Autodesk Inventor part; units mm, degrees
ref_plane "YZ Plane" through (0, 0, 0) normal (1, 0, 0) x (0, 1, 0)
ref_plane "XZ Plane" through (0, 0, 0) normal (0, 1, 0) x (-1, 0, 0)
ref_plane "XY Plane" through (0, 0, 0) normal (0, 0, 1) x (1, 0, 0)
sketch "Sketch1" plane through (0, 0, 0) normal (0, 1, 0) x (-1, 0, 0)
  line L0 (0, 0) -> (0, -3)
  line L1 (-250, -38) -> (-250, -78)
  line L2 (0, 0) -> (-20, 0)
  line L3 (-50, 0) -> (-50, -3)
  line L4 (-50, 0) -> (-70, 0)
  line L5 (-70, 0) -> (-70, -3)
  line L6 (-100, 0) -> (-100, -3)
  line L7 (-100, 0) -> (-120, 0)
  line L8 (-120, 0) -> (-120, -3)
  line L9 (-150, 0) -> (-150, -3)
  line L10 (-150, 0) -> (-170, 0)
  line L11 (-170, 0) -> (-170, -3)
  line L12 (-200, 0) -> (-200, -3)
  line L13 (-200, 0) -> (-220, 0)
  line L14 (-220, 0) -> (-220, -3)
  line L15 (-20, 0) -> (-20, -3)
  line L16 (-250, -58) -> (-250, -78)
  line L17 (-250, -78) -> (-247, -78)
  line L18 (-247, -78) -> (-247, -113)
  line L19 (-250, -58) -> (-250, -38)
  line L20 (-250, -38) -> (-247, -38)
  line L21 (-247, -38) -> (-247, -3)
  line L22 (-220, -3) -> (-247, -3)
  line L23 (-170, -3) -> (-200, -3)
  line L24 (-120, -3) -> (-150, -3)
  line L25 (-20, -3) -> (-50, -3)
  line L26 (-70, -3) -> (-100, -3)
  line L27 (0, -116) -> (0, -113)
  line L28 (0, -116) -> (-20, -116)
  line L29 (-50, -116) -> (-50, -113)
  line L30 (-50, -116) -> (-70, -116)
  line L31 (-70, -116) -> (-70, -113)
  line L32 (-100, -116) -> (-100, -113)
  line L33 (-100, -116) -> (-120, -116)
  line L34 (-120, -116) -> (-120, -113)
  line L35 (-150, -116) -> (-150, -113)
  line L36 (-150, -116) -> (-170, -116)
  line L37 (-170, -116) -> (-170, -113)
  line L38 (-200, -116) -> (-200, -113)
  line L39 (-200, -116) -> (-220, -116)
  line L40 (-220, -116) -> (-220, -113)
  line L41 (-20, -116) -> (-20, -113)
  line L42 (-3, -58) -> (-3, -78)
  line L43 (-3, -78) -> (0, -78)
  line L44 (-3, -58) -> (-3, -38)
  line L45 (-3, -38) -> (0, -38)
  line L46 (0, -113) -> (0, -78)
  line L47 (0, -38) -> (0, -3)
  line L48 (-50, -113) -> (-20, -113)
  line L49 (-100, -113) -> (-70, -113)
  line L50 (-150, -113) -> (-120, -113)
  line L51 (-247, -113) -> (-220, -113)
  line L52 (-200, -113) -> (-170, -113)
  line L53 (-53, -56) -> (-93, -56)
  line L54 (-93, -56) -> (-93, -53)
  line L55 (-93, -53) -> (-53, -53)
  line L56 (-53, -53) -> (-53, -56)
  line L57 (-197, -56) -> (-197, -53)
  line L58 (-197, -53) -> (-157, -53)
  line L59 (-157, -53) -> (-157, -56)
  line L60 (-157, -56) -> (-197, -56)
  dimension "d2" = 110
  dimension "d3" = 20
  dimension "d4" = 20
  dimension "d5" = 20
  dimension "d7" = 20
  dimension "d8" = 20
  dimension "d9" = 20
  dimension "d10" = 3
  dimension "d11" = 20
  dimension "d12" = 3
  dimension "d13" = 250
  dimension "d14" = 30
  dimension "d15" = 30
  dimension "d16" = 30
  dimension "d17" = 30
  dimension "d21" = 244
  dimension "d24" = 40
  dimension "d25" = 3
  dimension "d28" = 3
  dimension "d29" = 40
  dimension "d30" = 3
  dimension "d32" = 2
  dimension "d34" = 50
  dimension "d35" = 2
  dimension "d36" = 50
  dimension "d37" = 57
  dimension "d38" = 247
  dimension "d39" = 20
  dimension "d40" = 20
extrude "Extrusion2" add sketch "Sketch1" along normal blind 3
properties part number "latBack"
Verification items for the finished model (mm, model axes). Coordinates: 2 decimals unless noted, no trailing zeros. Order: outer loops, then holes, each group sorted by start corner. A loop starts at its lowest first (then second) coordinate and runs counter-clockwise, first axis right, second up. Notation, with made-up numbers: (40, 80.5) -> (44, 80.5) arc R9 ccw to (44, 93.5) -> close; hole circle Ø5 at (80, -25). An arc over 180 degrees is marked (long way). Put each result on its own line as item: value. Start each with the question number.
1. Cross-section at C-C, the plane x = 134. Record the boundary of the cut face in (y, z).
2. Go/stop test with flat-tipped pins: pin 1 Ø0.9 at (y, z) = (1.5, -2) entering from +X; pin 2 Ø0.9 at (x, y) = (78.5, 2) entering from +Z; pin 3 Ø1.5 at (x, y) = (84, 1.5) entering from -Z. Record where each tip stops, or that it passes through.
3. Cross-section at B-B, the plane y = 2.5. Count the separate pieces of the cut face and the enclosed holes in it, then the cut area to 3 significant figures.
4. Material ranges on L1, parallel to X at y = 1.05, z = -54.5; L2, parallel to Z at x = 68.5, y = 0.75; L3, parallel to Z at x = 22, y = 1.9, recorded low to high. Write a range as [from, to].
5. Cross-section at A-A, the plane x = 167. Record the boundary of the cut face in (y, z), then the cut area to 3 significant figures.
Computed:
1. outline: (0, -113) -> (3, -113) -> (3, -3) -> (0, -3) -> close
2. pin 1: x = 220
2. pin 2: z = -3
2. pin 3: z = -113
3. separate pieces: 1
3. enclosed holes: 2
3. area: 27,500 mm2
4. L1: [3, 53], [93, 157], [197, 250]
4. L2: [-116, -56], [-53, 0]
4. L3: [-113, -3]
5. outline: (0, -116) -> (3, -116) -> (3, -56) -> (0, -56) -> close; (0, -53) -> (3, -53) -> (3, 0) -> (0, 0) -> close
5. area: 339 mm2
